from build123d import *

# Parameters (mm, degrees)
BOSS_EXTRU_4_DEPTH = 5


with BuildPart() as part:
    # Esquisse1 → Boss.-Extru.4 (new body)
    with BuildSketch(Plane.XY):
        with BuildLine():
            Line((0, 0), (190.985155098, 0))
            ThreePointArc((190.985155098, 0), (193.599787646, -0.738111142), (195.442464428, -2.734521343))
            Line((195.442464428, -2.734521343), (193.518187839, -3.889087297))
            Line((193.518187839, -3.889087297), (177.22242063, -3.889087297))
            Line((177.22242063, -3.889087297), (3.889087297, -107.889087297))
            Line((3.889087297, -107.889087297), (3.889087297, -117.666547622))
            Line((3.889087297, -117.666547622), (2.58933145, -118.44640113))
            ThreePointArc((2.58933145, -118.44640113), (0.695737999, -116.610186592), (0, -114.065912899))
            Line((0, -114.065912899), (0, 0))
        make_face()
        Polygon((3.889087297, -102.889087297), (168.889087297, -3.889087297), (3.889087297, -3.889087297), align=None, mode=Mode.SUBTRACT)
    extrude(amount=BOSS_EXTRU_4_DEPTH)


solid = part.part
Geometry check sheet. Reference: the model listing, model coordinates, mm. A direction names the side the tool comes from. Give positions to 0.01 mm unless a question says otherwise; leave off trailing zeros. Loops run counter-clockwise (first coordinate to the right, second up) from the corner with the lowest first, then second, coordinate; pieces in that order, holes last. Notation, with made-up numbers: M 65.5,-20 L 82.5,-20 A12 ccw 82.5,-13 Z; hole C 3.5,48.25 d2. An arc over 180 degrees is marked long. Answer as a JSON object with one key per item and string values. Group by question number.
Item 1: Material ranges on L1, parallel to X at y = -88, z = 3.6; L2, parallel to Y at x = 30, z = 1.45; L3, parallel to X at y = -90, z = 2.25, recorded low to high.
Item 2: Gauge pin test, flat ends, axial feed: pin 1 (2.5 mm diameter, centred on y = -76.5, z = 1.5, fed in from +X); pin 2 (2 mm diameter, centred on x = 152, y = -20, fed in from -Z); pin 3 (1 mm diameter, centred on y = -25.5, z = 2.5, fed in from +X); pin 4 (2.5 mm diameter, centred on y = -112.5, z = 3.5, fed in from +X). Record the tip position at first contact, or that the pin passes through.
Item 3: Sectioned sample at A-A on z = 3.1. Record the boundary of the cut face in (x, y), plus the area to 3 significant figures.
Item 4: Sectioned sample at C-C on x = 69.5. Record the boundary of the cut face in (y, z).
Item 5: Mould release check, pull along Y, two halves, no side actions. Record for faces 1 (the flat face through (94, 0, 2)), 2 (the flat face through (105, -46, 5)), 3 (the flat face through (3.889, -53, 2)), 4 (the flat face through (85.234, -54.082, 2.465)): pulls with the +Y half, pulls with the -Y half, needs draft (parallel to the pull), parting line crosses it, or undercut.
Item 6: Access from +Z, -Z, +X, -X, +Y, -Y to the whole of each face (thin tool, end or side, straight path). Record for faces 5 (the flat face through (0, -58, 2)), 6 (the flat face through (88, -3.889, 2)), 7 (the flat face through (185, -3.889, 2)).
Item 7: Sectioned sample at B-B on y = -68. Record the boundary of the cut face in (x, z).
Findings below:
{
 "1": {"L1": "0 to 3.89, 28.7 to 37.04", "L2": "-92.22 to -87.22, -3.89 to 0", "L3": "0 to 3.89, 25.37 to 33.7"},
 "2": {"pin 1": "x = 58.29", "pin 2": "z = 0", "pin 3": "x = 142.04", "pin 4": "x = 3.89"},
 "3": {"outline": "M 0,-114.07 A5 ccw 2.59,-118.45 L 3.89,-117.67 L 3.89,-107.89 L 177.22,-3.89 L 193.52,-3.89 L 195.44,-2.73 A5 ccw 190.99,0 L 0,0 Z; hole M 3.89,-102.89 L 168.89,-3.89 L 3.89,-3.89 Z", "area": "2,040 mm2"},
 "4": {"outline": "M -68.52,0 L -63.52,0 L -63.52,5 L -68.52,5 Z; M -3.89,0 L 0,0 L 0,5 L -3.89,5 Z"},
 "5": {"face 1": "pulls with the +Y half", "face 2": "needs draft", "face 3": "undercut", "face 4": "undercut"},
 "6": {"face 5": "+Z, -Z, -X, +Y, -Y", "face 6": "+Z, -Z", "face 7": "+Z, -Z, +X, -Y"},
 "7": {"outline": "M 0,0 L 3.89,0 L 3.89,5 L 0,5 Z; M 62.04,0 L 70.37,0 L 70.37,5 L 62.04,5 Z"}
}
